Study the drawing (mm; zero at the part's minimum x, y, z) and answer. A direction names the side the tool comes from. Round coordinates to 2 decimals unless told otherwise and drop trailing zeros. Write each loop counter-clockwise with the first axis right and the second up, starting at its lowest first coordinate (ties: lowest second). Pieces come first, ordered by that corner, then holes. Notation, with made-up numbers: (26.5, 29.5) - (85.5, 29.5) arc R14 cw to (85.5, 42.5) - close; hole circle Ø7 at (-9.5, -0.5). An arc over 180 degrees is marked (long way). Use one line per item in the form item = value. Start each with the question number.
1) The part is cut by section C-C, the plane x = 97. Give the vertices of the cut face in (y, z), plus the area to 3 significant figures.
2) Each of these flat-tipped pins is pushed along its axis until it touches: pin 1 (1.5 mm diameter, centred on x = 77, y = 22, fed in from +Z); pin 2 (6 mm diameter, centred on y = 4.5, z = 13, fed in from +X); pin 3 (1 mm diameter, centred on x = 86.5, y = 5, fed in from -Z). Where does it stop, or does it pass through?
3) The part is cut by section D-D, the plane y = 5. Give the vertices of the cut face in (x, z).
4) Consider line 1 along Z through (x, y) = (3, 15); line 2 along Z through (x, y) = (50, 5.5); line 3 along X through (y, z) = (3.75, 7.5). Determine where each line is inside the solid, lowest interval first. Write a range as from..to.
5) For a pull along X with two mould halves and no side action, classify the marked faces 4 and 5 as released by +X, released by -X, zero draft, split by the parting line, or undercut.
6) The part is cut by section B-B, the plane y = 19. Give the vertices of the cut face in (x, z) (3 decimals).
7) For the marked faces 1, 2 and 3, determine the directions among +Z, -Z, +X, -X, +Y, -Y from which every point of the face is accessible in a straight line to the end or side of a thin tool.
8) The part is cut by section A-A, the plane z = 7.5. Give the vertices of the cut face in (x, y) (3 decimals), plus the area to 3 significant figures.
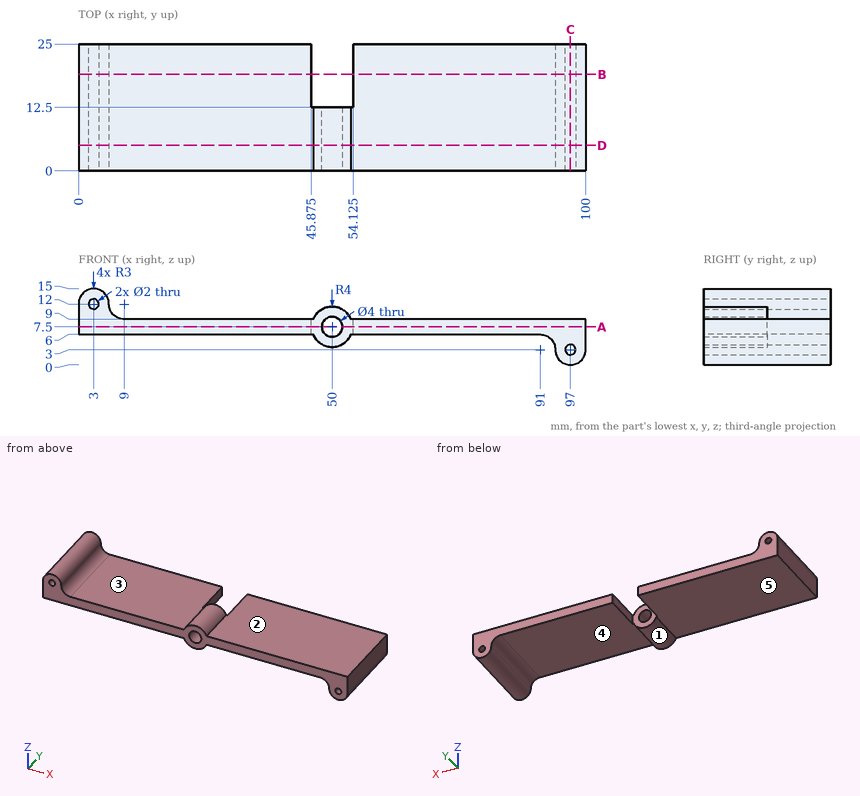
Geometry results:
q1.outline = (0, 0) - (25, 0) - (25, 2) - (0, 2) - close; (0, 4) - (25, 4) - (25, 9) - (0, 9) - close
q1.area = 175 mm2
q2.pin_1 = 9
q2.pin_2 = 53.12
q2.pin_3 = 6
q3.outline = (0, 6) - (46.29, 6) arc R4 ccw to (53.71, 6) - (91, 6) arc R3 cw to (94, 3) arc R3 ccw to (100, 3) - (100, 9) - (53.71, 9) arc R4 ccw to (46.29, 9) - (9, 9) arc R3 cw to (6, 12) arc R3 ccw to (0, 12) - close; hole circle Ø2 at (3, 12); hole circle Ø4 at (50, 7.5); hole circle Ø2 at (97, 3)
q4.line_1 = 6..11, 13..15
q4.line_2 = 3.5..5.5, 9.5..11.5
q4.line_3 = 0..48, 52..100
q5.face_4 = undercut
q5.face_5 = zero draft
q6.outline = (0, 6) - (45.875, 6) - (45.875, 9) - (9, 9) arc R3 cw to (6, 12) arc R3 ccw to (0, 12) - close; (54.125, 6) - (91, 6) arc R3 cw to (94, 3) arc R3 ccw to (100, 3) - (100, 9) - (54.125, 9) - close; hole circle Ø2 at (3, 12); hole circle Ø2 at (97, 3)
q7.face_1 = -Z, +Y, -Y
q7.face_2 = +Z, +X, +Y, -Y
q7.face_3 = +Z, +Y, -Y
q8.outline = (0, 0) - (48, 0) - (48, 12.5) - (45.875, 12.5) - (45.875, 25) - (0, 25) - close; (52, 0) - (100, 0) - (100, 25) - (54.125, 25) - (54.125, 12.5) - (52, 12.5) - close
q8.area = 2,350 mm2
